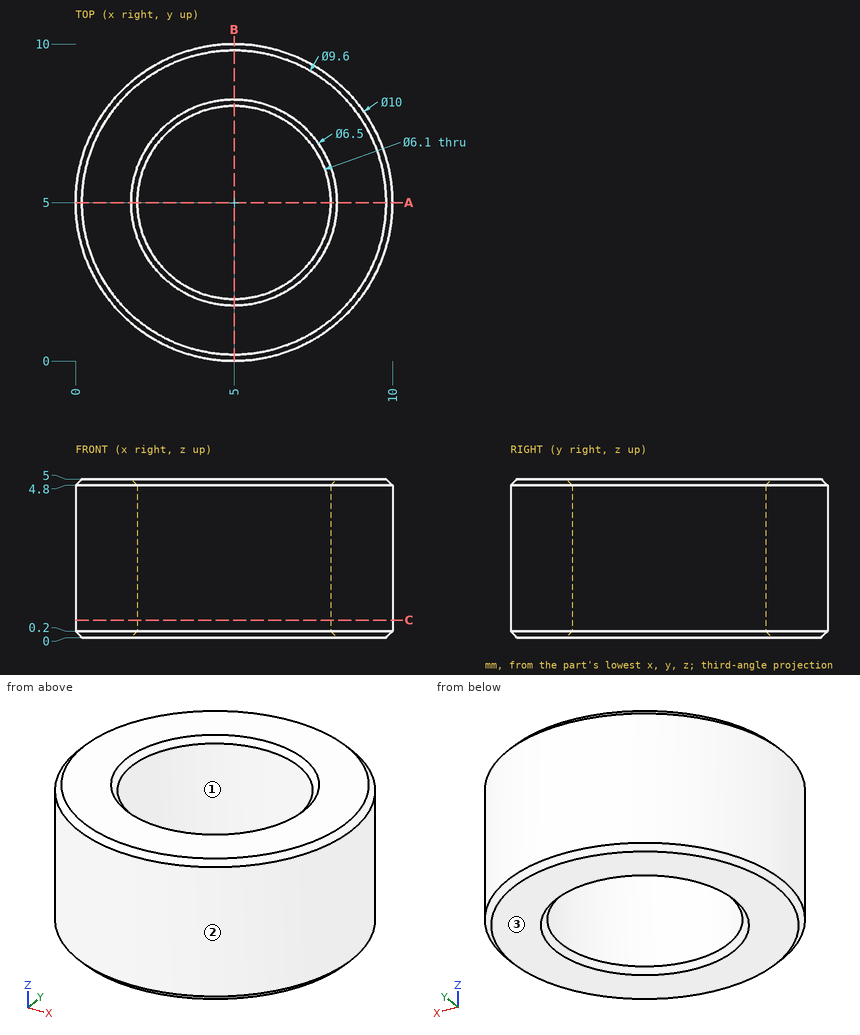
Answer from the drawing. Dimensions are ordinates in mm from the lowest x, y and z of the part. Give positions to 0.01 mm unless a question says otherwise; leave off trailing zeros. Write each loop counter-clockwise with the first axis right and the second up, starting at its lowest first coordinate (ties: lowest second). Pieces come first, ordered by that corner, then holes. Notation, with made-up numbers: M 53.25,-16.75 L 78.25,-16.75 A14 ccw 78.25,2.25 Z; hole C -20.5,53.5 d6. An arc over 180 degrees is marked long. Answer as CSV lines item,"result".
Q1. A cutting plane is placed at A-A on y = 5. Write down the section's boundary in (x, z), plus the area to 3 significant figures.
A:
outline,"M 0,0.2 L 0.2,0 L 1.75,0 L 1.95,0.2 L 1.95,4.8 L 1.75,5 L 0.2,5 L 0,4.8 Z; M 8.05,0.2 L 8.25,0 L 9.8,0 L 10,0.2 L 10,4.8 L 9.8,5 L 8.25,5 L 8.05,4.8 Z"
area,"19.3 mm²"
Q2. The mould has two halves that part along X. Classify the marked faces 1, 2 and 3: +X half, -X half, draft (parallel to the pull), parting line (faces both ways), or undercut.
A:
face 1,"undercut"
face 2,"parting line"
face 3,"draft"
Q3. Find the intervals of material crossed by probe 1 along Y at (x, z) = (5, 2.85); probe 2 along X at (y, z) = (2.75, 1.2); probe 3 along Y at (x, z) = (3.5, 4.75), in increasing order. Write a range as [from, to].
A:
probe 1,"y = [0, 1.95], [8.05, 10]"
probe 2,"x = [0.53, 2.94], [7.06, 9.47]"
probe 3,"y = [0.23, 2.34], [7.66, 9.77]"
Q4. A cutting plane is placed at C-C on z = 0.55. Write down the section's boundary in (x, y), plus the area to 3 significant figures.
A:
outline,"C 5,5 d10; hole C 5,5 d6.1"
area,"49.3 mm²"
Q5. Given P1, Ø1, axis at x = 6, y = 4, coming from the +Z side; P2, Ø1.5, axis at y = 7, z = 1, coming from the -X side, each flat-ended and moving along its own axis, determine where each tip first touches the part or whether it passes through.
A:
P1,"passes through"
P2,"stops at x = 0.16"
